Input: dimensioned drawing with shaded views. Units: mm. Origin: part minimum x, y, z. A direction names the side the tool comes from. Coordinates: 2 decimals unless noted, no trailing zeros. Order: outer loops, then holes, each group sorted by start corner. A loop starts at its lowest first (then second) coordinate and runs counter-clockwise, first axis right, second up. Notation, with made-up numbers: (42, -7) -> (54, -7) arc R13 cw to (54, 2) -> close; hole circle Ø2 at (75, -30). An arc over 180 degrees is marked (long way). Put each result on its own line as item: value.
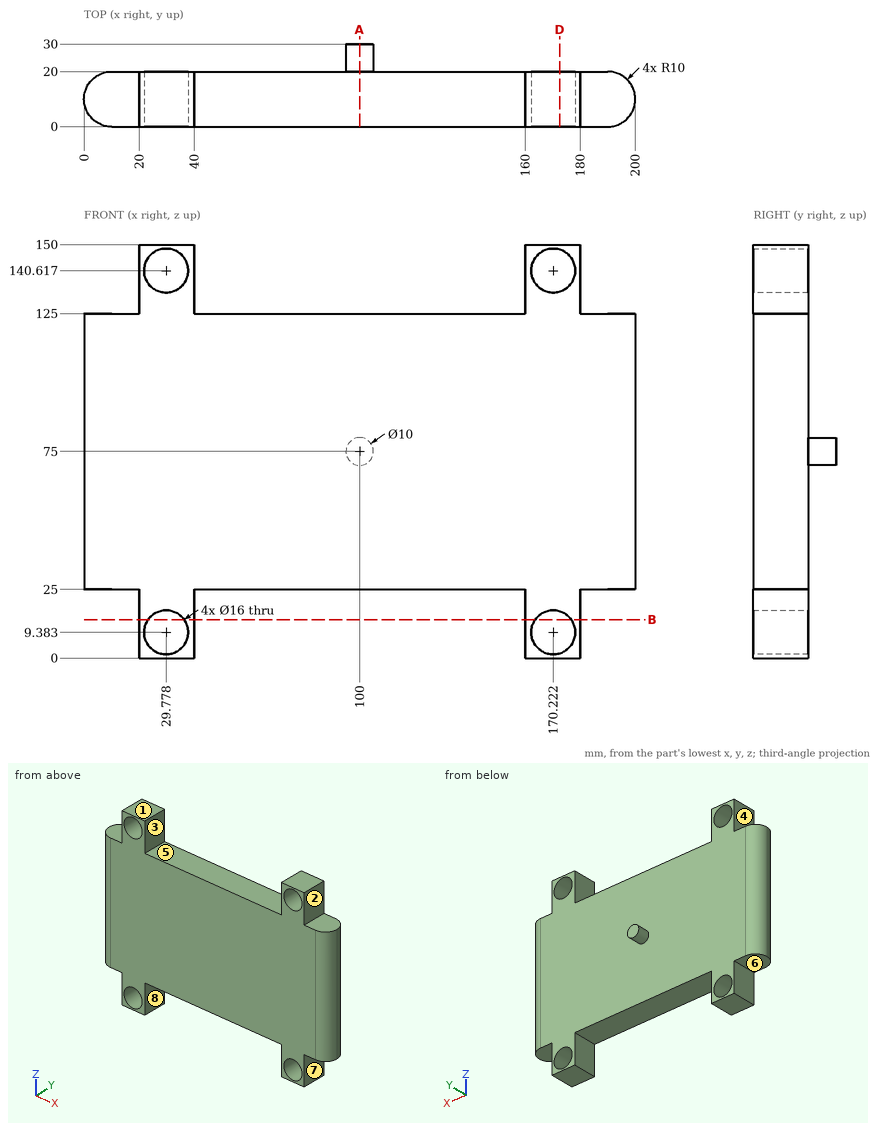
1. Set-up query: the marked faces 5, 6, 7 and 8. Return all of +Z, -Z, +X, -X, +Y, -Y with unobstructed straight access to the full face (end or side cutting, diameter ignored); none if empty.
Numbers:
face 5: +Z, +Y, -Y
face 6: -Z, -X, +Y, -Y
face 7: -Z, +X, +Y, -Y
face 8: -Z, +Y, -Y
2. First-contact query: pin 1 (6 mm diameter, centred on x = 100, y = 15.5, fed in from -Z); pin 2 (18.5 mm diameter, centred on x = 29.78, z = 140.62, fed in from +Y); pin 3 (6 mm diameter, centred on y = 5.5, z = 136, fed in from -X). Flat tips, straight axial feed; report the tip coordinate or a pass-through.
Numbers:
pin 1: stops at z = 25
pin 2: stops at y = 20
pin 3: stops at x = 20
3. Pull-direction query (X, two-part tool) for the marked faces 1, 2, 3 and 4; classes: pulls with the +X half, pulls with the -X half, needs draft (parallel to the pull), parting line crosses it, or undercut.
Numbers:
face 1: needs draft
face 2: pulls with the +X half
face 3: undercut
face 4: pulls with the -X half
4. Ray query, line 1 along X through (y, z) = (6, 141); line 2 along X through (y, z) = (6.5, 135) (1 decimal); line 3 along Z through (x, y) = (97.5, 17.5). Return the intervals inside material, ascending.
Numbers:
line 1: x = 20 to 21.79, 37.77 to 40, 160 to 162.23, 178.21 to 180
line 2: x = 20 to 24.1, 35.5 to 40, 160 to 164.5, 175.9 to 180
line 3: z = 25 to 125
5. Cut plane B-B on z = 14. Output: boundary loops of the cut face in (x, y) (1 decimal), plus the area to 3 significant figures.
Numbers:
outline: (20, 0) -> (23.2, 0) -> (23.2, 20) -> (20, 20) -> close; (36.3, 0) -> (40, 0) -> (40, 20) -> (36.3, 20) -> close; (160, 0) -> (163.7, 0) -> (163.7, 20) -> (160, 20) -> close; (176.8, 0) -> (180, 0) -> (180, 20) -> (176.8, 20) -> close
area: 277 mm2
6. Cut plane D-D on x = 172.5. Output: boundary loops of the cut face in (y, z) (1 decimal).
Numbers:
outline: (0, 0) -> (20, 0) -> (20, 1.7) -> (0, 1.7) -> close; (0, 17.1) -> (20, 17.1) -> (20, 132.9) -> (0, 132.9) -> close; (0, 148.3) -> (20, 148.3) -> (20, 150) -> (0, 150) -> close
7. Cut plane A-A on x = 100. Output: boundary loops of the cut face in (y, z).
Numbers:
outline: (0, 25) -> (20, 25) -> (20, 70) -> (30, 70) -> (30, 80) -> (20, 80) -> (20, 125) -> (0, 125) -> close
